Geometry: see drawing. Coordinates: mm, zero at the bounding-box minimum. Coordinates: 2 decimals unless noted, no trailing zeros. Write each loop counter-clockwise with the first axis right and the second up, starting at its lowest first coordinate (ties: lowest second). Pieces come first, ordered by that corner, then holes. Notation, with made-up numbers: (30.5, -36.5) -> (64.5, -36.5) arc R32 ccw to (64.5, -1.5) -> close; hole circle Ø3 at (-15, 52.5). An arc over 180 degrees is marked (long way). Use one line per item in the form item = value. Start each with the question number.
(1) Cut plane D-D on x = 37.5. Return the cut outline in (y, z), plus the area to 3 significant figures.
(2) Cut plane B-B on x = 3.69. Return the cut outline in (y, z).
(3) First-contact query: pin 1 (1 mm diameter, centred on x = 37, y = 12, fed in from -Z); pin 2 (0.6 mm diameter, centred on x = 29, z = 1, fed in from +Y). Flat tips, straight axial feed; report the tip coordinate or a pass-through.
(4) Cut plane A-A on y = 7.5. Return the cut outline in (x, z).
(5) Cut plane C-C on z = 1. Return the cut outline in (x, y) (1 decimal), plus the area to 3 significant figures.
(6) Ray query, line 1 along X through (y, z) = (7.5, 1.35); line 2 along Y through (x, z) = (35, 1); line 3 along Y through (x, z) = (4, 0.2). Return the intervals inside material, ascending.
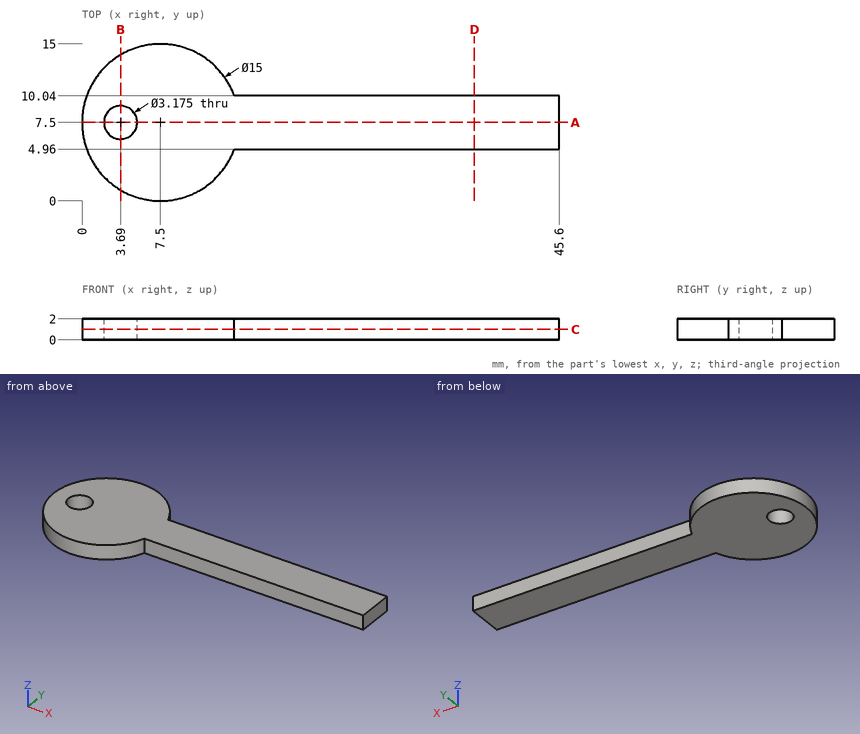
Values:
q1.outline = (4.96, 0) -> (10.04, 0) -> (10.04, 2) -> (4.96, 2) -> close
q1.area = 10.2 mm2
q2.outline = (1.04, 0) -> (5.91, 0) -> (5.91, 2) -> (1.04, 2) -> close; (9.09, 0) -> (13.96, 0) -> (13.96, 2) -> (9.09, 2) -> close
q3.pin_1 = through
q3.pin_2 = 10.04
q4.outline = (0, 0) -> (2.1, 0) -> (2.1, 2) -> (0, 2) -> close; (5.28, 0) -> (45.6, 0) -> (45.6, 2) -> (5.28, 2) -> close
q5.outline = (14.6, 5) -> (45.6, 5) -> (45.6, 10) -> (14.6, 10) arc R7.5 ccw (long way) to start; hole circle Ø3.2 at (3.7, 7.5)
q5.area = 325 mm2
q6.line_1 = 0 to 2.1, 5.28 to 45.6
q6.line_2 = 4.96 to 10.04
q6.line_3 = 0.87 to 5.94, 9.06 to 14.13
